Verification items for the finished model (mm, model axes). A direction names the side the tool comes from. Give positions to 0.01 mm unless a question says otherwise; leave off trailing zeros. Order: outer loops, then holes, each group sorted by start corner. A loop starts at its lowest first (then second) coordinate and runs counter-clockwise, first axis right, second up. Notation, with made-up numbers: (-3.75, 52) - (17.25, 52) arc R29 ccw to (17.25, 74) - close; hole circle Ø2 at (8.25, 53.25). An arc over 180 degrees is marked (long way). Answer as a JSON object with one key per item and string values.
```python
from build123d import *
from build123d.topology import SkipClean

# Parameters (mm, degrees)
SKETCH28_R           = 1.55
SKETCH28_R_2         = 4.5
SKETCH28_R_3         = 2
SKETCH28_W           = 10
SKETCH28_H           = 3
BOSS_EXTRUDE10_DEPTH = 5
SKETCH29_R           = 16
BOSS_EXTRUDE11_DEPTH = 2
SKETCH30_R           = 8.2
CUT_EXTRUDE1_DEPTH   = 5
SKETCH31_R           = 3.5
CUT_EXTRUDE2_DEPTH   = 3


with BuildPart() as part:
    # Sketch28 → Boss-Extrude10 (new body)
    with BuildSketch(Plane(origin=(-32, 0, 0), x_dir=(0, 0, 1), z_dir=(0, -1, 0))):
        with BuildLine():
            Line((-25, 15), (25, 15))
            Line((25, 15), (25, 5))
            Line((25, 5), (16, -145))
            ThreePointArc((16, -145), (0, -161), (-16, -145))
            Line((-16, -145), (-25, 5))
            Line((-25, 5), (-25, 15))
        make_face()
        with Locations(Location((8, 8.5, 0), (0, 0, 180))):
            Circle(SKETCH28_R, mode=Mode.SUBTRACT)
        with Locations(Location((-8, 8.5, 0), (0, 0, 180))):
            Circle(SKETCH28_R, mode=Mode.SUBTRACT)
        with Locations(Location((16, 11.5, 0), (0, 0, 180))):
            Circle(SKETCH28_R, mode=Mode.SUBTRACT)
        with Locations(Location((-16, 11.5, 0), (0, 0, 180))):
            Circle(SKETCH28_R, mode=Mode.SUBTRACT)
        with Locations(Location((-15.5, -6, 0), (0, 0, 180))):
            Circle(SKETCH28_R, mode=Mode.SUBTRACT)
        with Locations(Location((15.5, -6, 0), (0, 0, 180))):
            Circle(SKETCH28_R, mode=Mode.SUBTRACT)
        with Locations(Location((0, -65.5, 0), (0, 0, 180))):
            Circle(SKETCH28_R_2, mode=Mode.SUBTRACT)
        with Locations(Location((0, -20, 0), (0, 0, 180))):
            Circle(SKETCH28_R_3, mode=Mode.SUBTRACT)
        with Locations(Location((0, -145, 0), (0, 0, 180))):
            Circle(SKETCH28_R_2, mode=Mode.SUBTRACT)
        with Locations(Location((-9, -20, 0), (0, 0, 180))):
            Circle(SKETCH28_R, mode=Mode.SUBTRACT)
        with Locations(Location((0, -11, 0), (0, 0, 180))):
            Circle(SKETCH28_R, mode=Mode.SUBTRACT)
        with Locations(Location((9, -20, 0), (0, 0, 180))):
            Circle(SKETCH28_R, mode=Mode.SUBTRACT)
        with Locations(Location((0, -29, 0), (0, 0, 180))):
            Circle(SKETCH28_R, mode=Mode.SUBTRACT)
        with Locations((0, -4.5)):
            Rectangle(SKETCH28_W, SKETCH28_H, mode=Mode.SUBTRACT)
    extrude(amount=BOSS_EXTRUDE10_DEPTH)

    # Sketch29 → Boss-Extrude11 (add)
    with SkipClean():  # the faces are left unmerged after this step: merging them gives an invalid solid
        with BuildSketch(Plane.XZ.offset(5)):
            with Locations(Location((33.5, 0, 0), (0, 0, 270))):
                Circle(SKETCH29_R)
            with Locations(Location((113, 0, 0), (0, 0, 270))):
                Circle(SKETCH29_R)
        extrude(amount=BOSS_EXTRUDE11_DEPTH)
    add(part.part.scale(1), mode=Mode.REPLACE)  # the faces are merged on a copy

    # Sketch30 → Cut-Extrude1 (cut)
    with BuildSketch(Plane.XZ.offset(7)):
        with Locations(Location((33.5, 0, 0), (0, 0, 270))):
            Circle(SKETCH30_R)
        with Locations(Location((113, 0, 0), (0, 0, 270))):
            Circle(SKETCH30_R)
    extrude(amount=-CUT_EXTRUDE1_DEPTH, mode=Mode.SUBTRACT)

    # Sketch31 → Cut-Extrude2 (cut)
    with BuildSketch(Plane(origin=(0, 0, 0), x_dir=(1, 0, 0), z_dir=(0, 1, 0))):
        with Locations(Location((-12, 9, 0), (0, 0, 270))):
            Circle(SKETCH31_R)
        with Locations(Location((-3, 0, 0), (0, 0, 270))):
            Circle(SKETCH31_R)
        with Locations(Location((-12, -9, 0), (0, 0, 270))):
            Circle(SKETCH31_R)
        with Locations(Location((-21, 0, 0), (0, 0, 270))):
            Circle(SKETCH31_R)
    extrude(amount=-CUT_EXTRUDE2_DEPTH, mode=Mode.SUBTRACT)


solid = part.part
```
(1) Section check D-D (x = 99.5). Record the cut outline in (y, z).
Computed values:
{"outline": "(-7, -8.59) - (-5, -8.59) - (-5, -16.81) - (0, -16.81) - (0, 16.81) - (-5, 16.81) - (-5, 8.59) - (-7, 8.59) - close"}
(2) Access from +Z, -Z, +X, -X, +Y, -Y to the whole of each face (thin tool, end or side, straight path). Record for faces 1 (the flat face through (106, -7, -7)), 2 (the flat face through (-22, -3, 2)), 3 (the cylindrical face through (17.88, -5.99, 3.47)).
Computed values:
{"face 1": "+Z, -Z, +X, -X, -Y", "face 2": "+Y", "face 3": "-Y"}
(3) Material ranges on line 1 along X through (y, z) = (-4.25, -9); line 2 along Y through (x, z) = (47, -11); line 3 along X through (y, z) = (-6, 3), recorded low to high. Write a range as [from, to].
Computed values:
{"line 1": "x = [-47, -41.68], [-39.32, -13.55], [-10.45, 126.23]", "line 2": "y = [-5, 0]", "line 3": "x = [17.78, 25.87], [41.13, 49.22], [97.28, 105.37], [120.63, 128.72]"}
(4) Section check B-B (z = 0). Count the separate pieces of the cut face and the enclosed holes in it, then the cut area to 3 significant figures.
Computed values:
{"separate pieces": "7", "enclosed holes": "0", "area": "719 mm²"}
(5) Section check A-A (x = -3). Record the cut outline in (y, z).
Computed values:
{"outline": "(-5, -22.96) - (0, -22.96) - (0, -3.5) - (-3, -3.5) - (-3, -1.55) - (-5, -1.55) - close; (-5, 1.55) - (-3, 1.55) - (-3, 3.5) - (0, 3.5) - (0, 22.96) - (-5, 22.96) - close"}
(6) Release check for a two-part mould opening along X. For faces 4 (the cylindrical face through (-13.513, -3.986, -8.664)), 5 (the flat face through (41, -7, 4)), 6 (the cylindrical face through (-12.94, -3.99, 10.23)), 7 (the flat face through (-47, -2, 0)) record: pulls with the +X half, pulls with the -X half, needs draft (parallel to the pull), parting line crosses it, or undercut.
Computed values:
{"face 4": "undercut", "face 5": "needs draft", "face 6": "undercut", "face 7": "pulls with the -X half"}
(7) Section check C-C (x = 33.5). Record the cut outline in (y, z), then the cut area to 3 significant figures.
Computed values:
{"outline": "(-7, -16) - (-5, -16) - (-5, -20.77) - (0, -20.77) - (0, -4.5) - (-2, -4.5) - (-2, -8.2) - (-7, -8.2) - close; (-7, 8.2) - (-2, 8.2) - (-2, 4.5) - (0, 4.5) - (0, 20.77) - (-5, 20.77) - (-5, 16) - (-7, 16) - close", "area": "172 mm²"}
(8) Gauge pin test, flat ends, axial feed: pin 1 Ø2 at (x, z) = (-1.5, -1) entering from +Y; pin 2 Ø4 at (x, y) = (83.5, -4) entering from -Z; pin 3 Ø1.5 at (x, y) = (58, -4.5) entering from +Z (3 decimals); pin 4 Ø1.9 at (x, z) = (-26, -15.5) entering from +Y. Record the tip position at first contact, or that the pin passes through.
Computed values:
{"pin 1": "stops at y = -3", "pin 2": "stops at z = -17.89", "pin 3": "stops at z = 19.345", "pin 4": "passes through"}
